The figure shows three views and two pictorial views of one solid part (mm, origin at its lowest corner). Answer the questions. A direction names the side the tool comes from. Coordinates: 2 decimals unless noted, no trailing zeros. Loops run counter-clockwise (first coordinate to the right, second up) from the corner with the lowest first, then second, coordinate; pieces in that order, holes last. Notation, with made-up numbers: (-30, 13) - (21, 13) arc R16 ccw to (21, 34) - close; hole circle Ø4 at (82, 43). An arc over 180 degrees is marked (long way). Return JSON: item names as keys, results as strings. Group by question number.
1. Which of the six approach directions +Z, -Z, +X, -X, +Y, -Y give full straight-line access (tool end or side, diameter ignored) to the marked faces 4 and 5?
2. Section B-B (x = 54) is taken. Write down the section's boundary in (y, z) (1 decimal).
3. The mould has two halves that part along Z. Classify the marked faces 1, 2 and 3: pulls with the +Z half, pulls with the -Z half, needs draft (parallel to the pull), parting line crosses it, or undercut.
4. Section A-A (z = 135.5) is taken. Write down the section's boundary in (x, y) (1 decimal).
5. Section D-D (x = 123.5) is taken. Write down the section's boundary in (y, z), and give its area (3 significant figures).
6. Each of these flat-tipped pins is pushed along its axis until it touches: P1, Ø1, axis at x = 123, y = 10.5, coming from the +Z side (1 decimal); P2, Ø10, axis at y = 10.5, z = 163.5, coming from the +X side (1 decimal); P3, Ø2, axis at y = 20.5, z = 180, coming from the +X side. Where does it stop, or does it pass through?
7. Find the intervals of material crossed by line 1 along X through (y, z) = (19.75, 121) (1 decimal); line 2 along Z through (x, y) = (65.5, 1.5) (1 decimal); line 3 along Z through (x, y) = (44, 22), in increasing order.
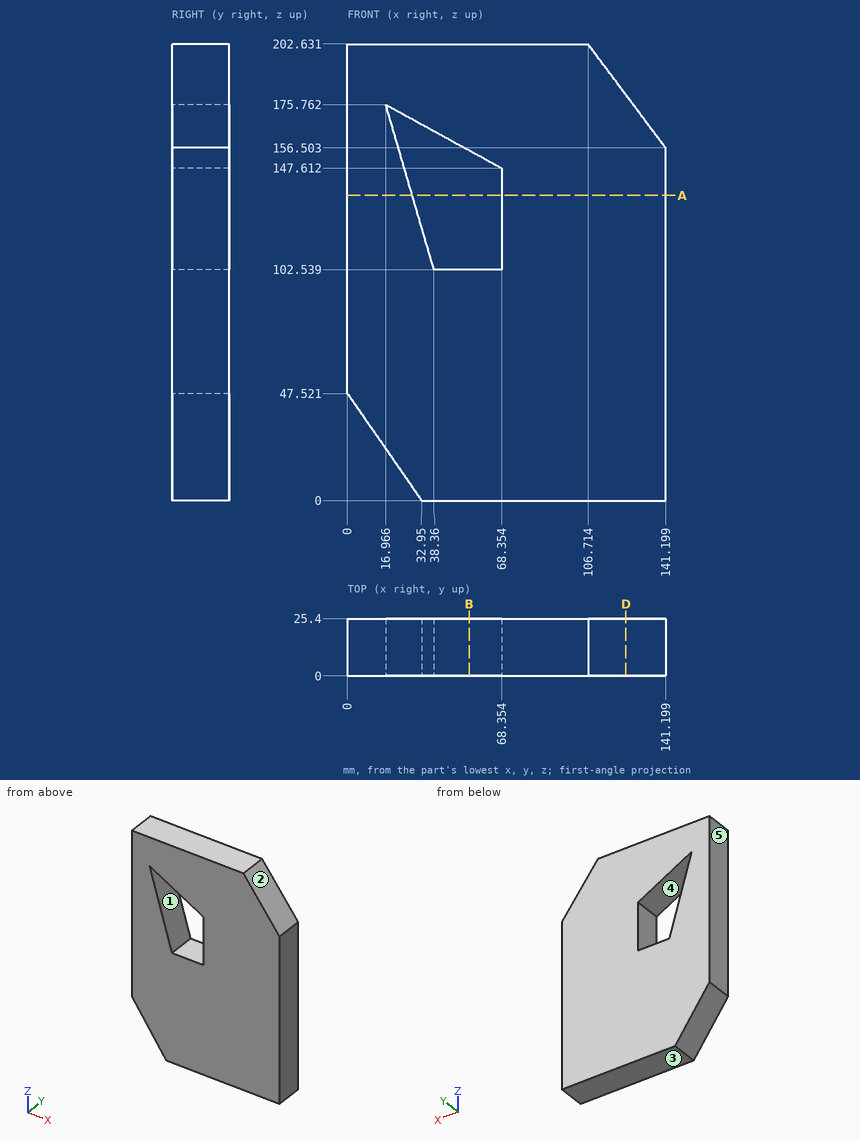
The answers:
{
 "1": {"face 4": "+Y, -Y", "face 5": "+Z, -Z, -X, +Y, -Y"},
 "2": {"outline": "(0, 0) - (25.4, 0) - (25.4, 102.5) - (0, 102.5) - close; (0, 155.5) - (25.4, 155.5) - (25.4, 202.6) - (0, 202.6) - close"},
 "3": {"face 1": "undercut", "face 2": "pulls with the +Z half", "face 3": "pulls with the -Z half"},
 "4": {"outline": "(0, 0) - (28.7, 0) - (28.7, 25.4) - (0, 25.4) - close; (68.4, 0) - (141.2, 0) - (141.2, 25.4) - (68.4, 25.4) - close"},
 "5": {"outline": "(0, 0) - (25.4, 0) - (25.4, 180.18) - (0, 180.18) - close", "area": "4,580 mm2"},
 "6": {"P1": "stops at z = 181.5", "P2": "stops at x = 139.7", "P3": "stops at x = 124.38"},
 "7": {"line 1": "x = 0 to 33, 68.4 to 141.2", "line 2": "z = 0 to 102.5, 149.2 to 202.6", "line 3": "z = 0 to 102.54, 160.95 to 202.63"}
}
